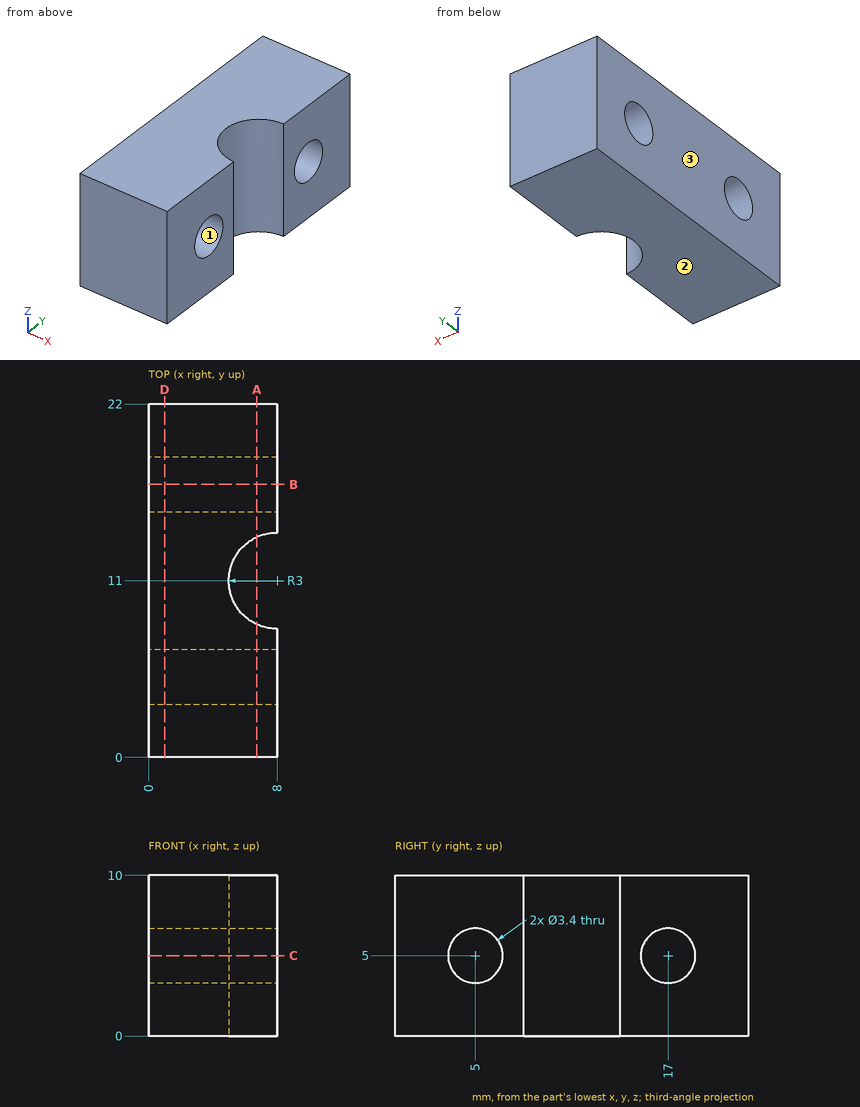
Can you work these out from the drawing? Everything is in mm from the part's minimum corner. Round coordinates to 2 decimals unless told otherwise and drop trailing zeros. Write each loop counter-clockwise with the first axis right and the second up, starting at its lowest first coordinate (ties: lowest second). Pieces come first, ordered by that corner, then holes. Notation, with made-up numbers: (35, -19.5) - (83, -19.5) arc R10 cw to (83, -1.5) - close; hole circle Ø9 at (34.25, -19.75). An arc over 180 degrees is marked (long way). Write each question's results on one line, items separated by ' | '. Start each with the question number.
1) Suppose I cut it at C-C (z = 5). List the corners of the cut face in (x, y) for me, and give its area (3 significant figures).
2) Suppose I cut it at B-B (y = 17). List the corners of the cut face in (x, z) for me.
3) Suppose I cut it at A-A (x = 6.75). List the corners of the cut face in (y, z) for me.
4) We'd pull the mould along Z, two halves only. Please class the marked faces 1, 2 and 3: released by +Z, released by -Z, zero draft, split by the parting line, or undercut.
5) Please list where these lines run through material, in increasing order: line 1 (Z direction, x = 6, y = 17); line 2 (Y direction, x = 0.5, z = 6.5); line 3 (Y direction, x = 2, z = 3.75).
6) Suppose I cut it at D-D (x = 1). List the corners of the cut face in (y, z) for me, and give its area (3 significant figures).
Here are the results:
1) outline: (0, 0) - (8, 0) - (8, 3.3) - (0, 3.3) - close; (0, 6.7) - (8, 6.7) - (8, 8) arc R3 cw to (8, 14) - (8, 15.3) - (0, 15.3) - close; (0, 18.7) - (8, 18.7) - (8, 22) - (0, 22) - close | area: 107 mm2
2) outline: (0, 0) - (8, 0) - (8, 3.3) - (0, 3.3) - close; (0, 6.7) - (8, 6.7) - (8, 10) - (0, 10) - close
3) outline: (0, 0) - (8.27, 0) - (8.27, 10) - (0, 10) - close; (13.73, 0) - (22, 0) - (22, 10) - (13.73, 10) - close; hole circle Ø3.4 at (5, 5); hole circle Ø3.4 at (17, 5)
4) face 1: undercut | face 2: released by -Z | face 3: zero draft
5) line 1: z = 0 to 3.3, 6.7 to 10 | line 2: y = 0 to 4.2, 5.8 to 16.2, 17.8 to 22 | line 3: y = 0 to 3.85, 6.15 to 15.85, 18.15 to 22
6) outline: (0, 0) - (22, 0) - (22, 10) - (0, 10) - close; hole circle Ø3.4 at (5, 5); hole circle Ø3.4 at (17, 5) | area: 202 mm2
